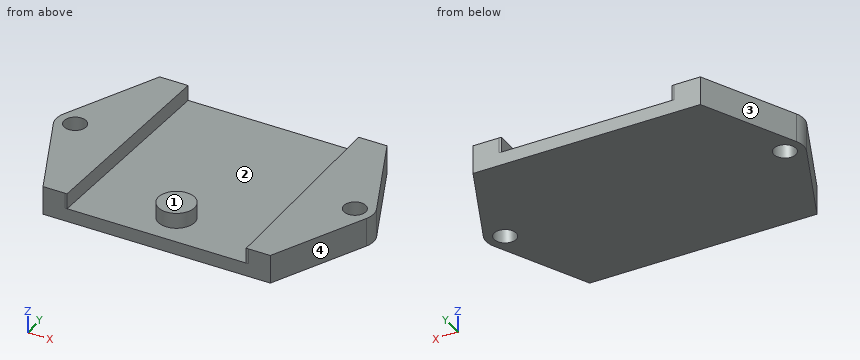
from build123d import *

# Parameters (mm, degrees)
F0_R     = 2.5
F0_R_2   = 4.125
F1_DEPTH = 6.5
F2_DEPTH = 3.5
F3_R     = 5
F4_DEPTH = 0.5
F5_DEPTH = 0.5


# Not quite as in the source:
# - a feature names something its author has since deleted; it is built from what else it names


with BuildPart() as f1:
    # F0 (on Top) → F1 (new body)
    with BuildSketch(Plane.XY):
        Polygon((-16.7020111382, 19.4748209119), (-22.7020111382, 19.4748209119), (-33.4520111382, -4.0251790881), (-22.7020111382, -27.5251790881), (-17.7020111382, -27.5251790881), align=None)
        with Locations((-28.7020111382, -4.0251790881)):
            Circle(F0_R, mode=Mode.SUBTRACT)
        Polygon((23.2979888618, 19.4748209119), (-16.7020111382, 19.4748209119), (-17.7020111382, -27.5251790881), (24.2979888618, -27.5251790881), align=None)
        with Locations((3.2979888618, -19.5251790881)):
            Circle(F0_R_2, mode=Mode.SUBTRACT)
        Polygon((29.2979888618, 19.4748209119), (23.2979888618, 19.4748209119), (24.2979888618, -27.5251790881), (29.2979888618, -27.5251790881), (40.0479888618, -4.0251790881), align=None)
        with Locations((35.2979888618, -4.0251790881)):
            Circle(F0_R, mode=Mode.SUBTRACT)
        with Locations((3.2979888618, -19.5251790881)):
            Circle(F0_R_2)
    extrude(amount=-F1_DEPTH)

    # F0 (on Top) → F2 (cut)
    with BuildSketch(Plane.XY):
        Polygon((23.2979888618, 19.4748209119), (-16.7020111382, 19.4748209119), (-17.7020111382, -27.5251790881), (24.2979888618, -27.5251790881), align=None)
        with Locations((3.2979888618, -19.5251790881)):
            Circle(F0_R_2, mode=Mode.SUBTRACT)
    extrude(amount=-F2_DEPTH, mode=Mode.SUBTRACT)

    # F3
    f3_edges = [f1.edges().sort_by_distance(p)[0] for p in [
        (-33.452011, -4.025179, -3.25),
        (40.047989, -4.025179, -3.25),
    ]]
    fillet(f3_edges, radius=F3_R)

    # F4 (add): a face of the model
    f4_faces = [f1.faces().sort_by_distance(p)[0] for p in [
        (-17.2020111382, -4.0251790881, -1.75),
    ]]
    extrude(f4_faces, amount=F4_DEPTH)

    # F5 (add): a face of the model
    f5_faces = [f1.faces().sort_by_distance(p)[0] for p in [
        (23.7979888618, -4.0251790881, -1.75),
    ]]
    extrude(f5_faces, amount=F5_DEPTH)


solid = f1.part
For this review, take the finished solid that the model builds, in its own axes (mm). Face numbers are marked on the shaded views. Round coordinates to 2 decimals unless told otherwise and drop trailing zeros. Write each loop counter-clockwise with the first axis right and the second up, starting at its lowest first coordinate (ties: lowest second). Pieces come first, ordered by that corner, then holes. Notation, with made-up numbers: M -11.5,-13.5 L 2.5,-13.5 A16 ccw 2.5,5.5 Z; hole C 32,53.25 d3. An arc over 180 degrees is marked long. Write item = value, one per line. Start each with the question number.
(1) The part is to be moulded in two halves that separate along X. For the marked faces 1, 2, 3 and 4, say which applies: +X half, -X half, draft (parallel to the pull), parting line (faces both ways), or undercut.
(2) We need section D-D (y = 9). Give the boundary of the cut face in (x, z), then the cut area to 3 significant figures.
(3) We need section C-C (x = 9.5). Give the boundary of the cut face in (y, z).
(4) We need section B-B (y = 15). Give the boundary of the cut face in (x, z).
(5) We need section A-A (z = -2.75). Give the boundary of the cut face in (x, y) (3 decimals).
(6) Clearance check with a flat-ended pin moving along its axis: pin 1 Ø3 at (x, y) = (-14, 0) entering from +Z. State where the tip first meets the part, or that it passes through.
(7) For line 1 along X through (y, z) = (-23, -1.25); line 2 along Y through (x, z) = (-20, -3); line 3 along X through (y, z) = (-14.5, -3), list the stretches that pass through material, from the lowest coordinate up.
Results found:
q1.face_1 = draft
q1.face_2 = undercut
q1.face_3 = -X half
q1.face_4 = +X half
q2.outline = M -27.49,-6.5 L 34.09,-6.5 L 34.09,0 L 23.02,0 L 23.02,-3.5 L -16.42,-3.5 L -16.42,0 L -27.49,0 Z
q2.area = 262 mm²
q3.outline = M -27.53,-6.5 L 19.47,-6.5 L 19.47,-3.5 L -27.53,-3.5 Z
q4.outline = M -24.75,-6.5 L 31.34,-6.5 L 31.34,0 L 22.89,0 L 22.89,-3.5 L -16.3,-3.5 L -16.3,0 L -24.75,0 Z
q5.outline = M -32.501,-6.105 L -22.702,-27.525 L -17.702,-27.525 L -17.202,-27.536 L -16.202,19.464 L -16.702,19.475 L -22.702,19.475 L -32.501,-1.945 A5 ccw Z; C 3.298,-19.525 d8.25; M 22.798,19.464 L 23.798,-27.536 L 24.298,-27.525 L 29.298,-27.525 L 39.097,-6.105 A5 ccw 39.097,-1.945 L 29.298,19.475 L 23.298,19.475 Z; hole C -28.702,-4.025 d5; hole C 35.298,-4.025 d5
q6.pin_1 = -3.5
q7.line_1 = -24.77 to -17.11, 1.08 to 5.52, 23.7 to 31.37
q7.line_2 = -27.53 to 19.47
q7.line_3 = -28.66 to -16.92, 23.52 to 35.26
